Here's the drawing with two shaded views (mm, measured from the low corner). I have some questions. Coordinates: 2 decimals unless noted, no trailing zeros. Write each loop counter-clockwise with the first axis right and the second up, starting at its lowest first coordinate (ties: lowest second). Pieces come first, ordered by that corner, then holes. Notation, with made-up numbers: (47.25, 69) -> (97.25, 69) arc R20 cw to (97.25, 73) -> close; hole circle Ø10 at (63.5, 81). An arc over 180 degrees is marked (long way). Use one line per item in the form item = value.
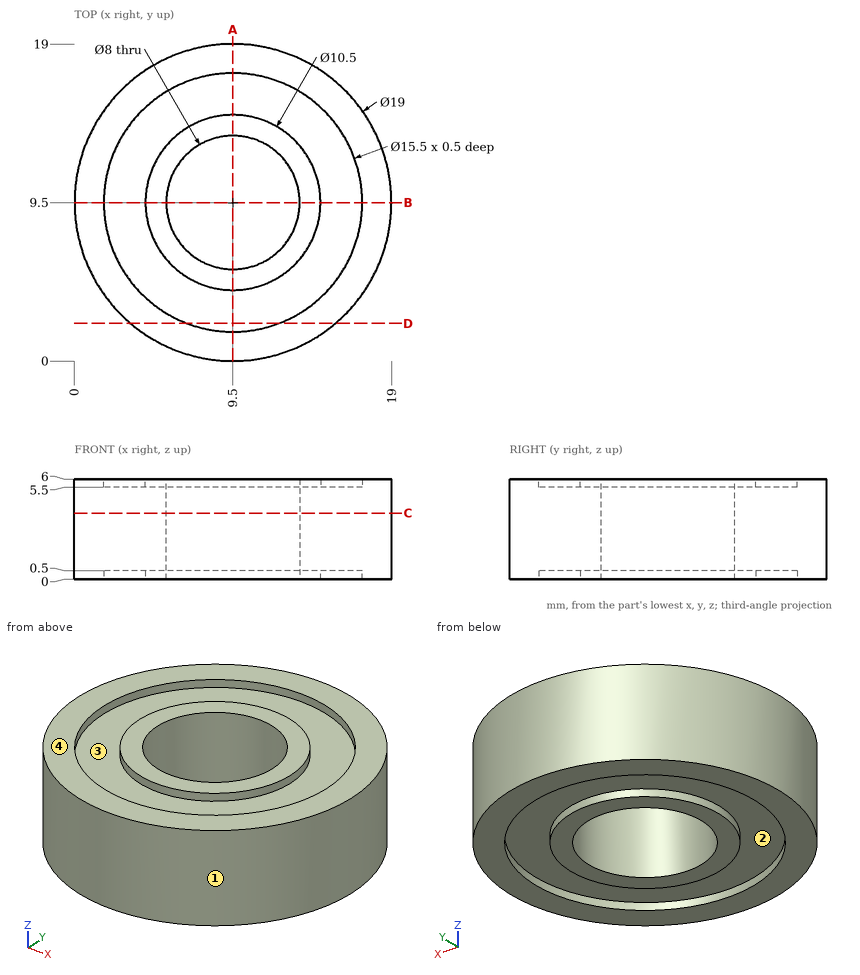
Q1. Suppose I cut it at A-A (x = 9.5). Write out the boundary of the cut face in (y, z).
Return value:
outline = (0, 0) -> (1.75, 0) -> (1.75, 0.5) -> (4.25, 0.5) -> (4.25, 0) -> (5.5, 0) -> (5.5, 6) -> (4.25, 6) -> (4.25, 5.5) -> (1.75, 5.5) -> (1.75, 6) -> (0, 6) -> close; (13.5, 0) -> (14.75, 0) -> (14.75, 0.5) -> (17.25, 0.5) -> (17.25, 0) -> (19, 0) -> (19, 6) -> (17.25, 6) -> (17.25, 5.5) -> (14.75, 5.5) -> (14.75, 6) -> (13.5, 6) -> close
Q2. Suppose I cut it at D-D (y = 2.25). Write out the boundary of the cut face in (x, z).
Return value:
outline = (3.36, 0) -> (6.76, 0) -> (6.76, 0.5) -> (12.24, 0.5) -> (12.24, 0) -> (15.64, 0) -> (15.64, 6) -> (12.24, 6) -> (12.24, 5.5) -> (6.76, 5.5) -> (6.76, 6) -> (3.36, 6) -> close
Q3. Suppose I cut it at C-C (z = 3.95). Write out the boundary of the cut face in (x, y), then the cut area to 3 significant figures.
Return value:
outline = circle Ø19 at (9.5, 9.5); hole circle Ø8 at (9.5, 9.5)
area = 233 mm2
Q4. Will this pin go through, and if not, where does the flat tip stop? pin 1 (1 mm diameter, centred on x = 16.5, z = 2, fed in from +Y).
Return value:
pin_1 = 16.43
Q5. If I drill on line 1 (Y direction, x = 9.5, z = 0.15); line 2 (Z direction, x = 7.75, y = 15.25); line 3 (Y direction, x = 9.5, z = 3.45), over which ranges is the centre line in solid material (lowest first)? Write a range as from..to.
Return value:
line_1 = 0..1.75, 4.25..5.5, 13.5..14.75, 17.25..19
line_2 = 0.5..5.5
line_3 = 0..5.5, 13.5..19
Q6. Thinking about a two-plate mould opening in X: for the marked faces 1, 2, 3 and 4, which applies, released by +X, released by -X, zero draft, split by the parting line, or undercut?
Return value:
face_1 = split by the parting line
face_2 = undercut
face_3 = undercut
face_4 = zero draft
